Read the model definition and answer for the solid it produces. Units are mm, in the model's axes. A direction names the side the tool comes from. Give positions to 0.01 mm unless a question says otherwise; leave off trailing zeros. Order: outer loops, then holes, each group sorted by start corner. A loop starts at its lowest first (then second) coordinate and runs counter-clockwise, first axis right, second up. Notation, with made-up numbers: (30, 68) - (75, 68) arc R24 cw to (75, 90) - close; hole circle Ø1 at (-9, 30). An arc over 180 degrees is marked (long way). Use a Markdown table: item, result. Add a question column.
1. Consider L1, parallel to Y at x = 4.4, z = 0; L2, parallel to X at y = 9.75, z = 2.5; L3, parallel to Y at x = 13.6, z = 0. Determine where each line is inside the solid, lowest interval first.
2. A cutting plane is placed at B-B on x = -112.5. Determine the outline of the cut face in (y, z).
3. For a pull along X with two mould halves and no side action, classify faces 6 (the cylindrical face through (2.769, 12.082, 5.323)), 7 (the cylindrical face through (-3.4, 19.3, -0.1)), 8 (the flat face through (12, 10, -4.648)) as released by +X, released by -X, zero draft, split by the parting line, or undercut.
4. Flat-ended cylindrical pins translate along their axes: P1, Ø1.5, axis at x = -109.5, y = 2, coming from the -Z side; P2, Ø0.7, axis at x = 2.5, y = 12.5, coming from the +Z side; P3, Ø3.5, axis at x = -79.5, z = 1, coming from the +Y side; P4, Ø6.5, axis at x = 7.5, z = 0.5, coming from the +Y side. Find the tip coordinate at first contact, or state that the pin passes through.
5. Which of the six approach directions +Z, -Z, +X, -X, +Y, -Y give full straight-line access (tool end or side, diameter ignored) to faces 1 (the flat face through (0, 18.551, 0)), 2 (the flat face through (12, 10, 4.638)), 3 (the flat face through (-75, 9, 5.764)), 4 (the flat face through (11.063, 8, 0)), 5 (the cylindrical face through (13.25, 12.22, -0.26))?
6. A cutting plane is placed at A-A on z = 0. Determine the outline of the cut face in (x, y).
```python
from build123d import *

# Parameters (mm, degrees)
SKETCH1_R               = 6
BOSS_EXTRUDE1_DEPTH     = 20
SKETCH2_R               = 3.4
CUT_EXTRUDE1_DEPTH      = 13.55
SKETCH5_W               = 1.550685087
SKETCH5_H               = 7.184215806
BOSS_EXTRUDE2_DEPTH     = 13.55
SKETCH7_W               = 9.286501956
SKETCH7_H               = 19.909960041
BOSS_EXTRUDE3_DEPTH     = 12.9
SKETCH6_R               = 2
CUT_EXTRUDE2_DEPTH      = 1
CUT_EXTRUDE2_DEPTH_BACK = 13.55
CUT_EXTRUDE3_DEPTH      = 10
CUT_EXTRUDE3_DEPTH_BACK = 10
SKETCH11_W              = 11.756176319
SKETCH11_H              = 18.551417714
BOSS_EXTRUDE4_DEPTH     = 153


with BuildPart() as part:
    # Sketch1 → Boss-Extrude1 (new body)
    with BuildSketch(Plane(origin=(0, 0, 0), x_dir=(1, 0, 0), z_dir=(0, 1, 0))):
        Circle(SKETCH1_R)
    extrude(amount=BOSS_EXTRUDE1_DEPTH)

    # Sketch2 → Cut-Extrude1 (cut)
    with BuildSketch(Plane(origin=(0, 20, 0), x_dir=(1, 0, 0), z_dir=(0, 1, 0))):
        Circle(SKETCH2_R)
    extrude(amount=-CUT_EXTRUDE1_DEPTH, mode=Mode.SUBTRACT)

    # Sketch5 → Boss-Extrude2 (add)
    with BuildSketch(Plane(origin=(0, 18.26, 0), x_dir=(1, 0, 0), z_dir=(0, 1, 0))):
        with Locations((3.375342544, 0.020519704)):
            Rectangle(SKETCH5_W, SKETCH5_H)
    extrude(amount=-BOSS_EXTRUDE2_DEPTH)

    # Sketch7 → Boss-Extrude3 (add)
    with BuildSketch(Plane.ZY.offset(-2.6)):
        with Locations((-0.005218197, 9.954980021)):
            Rectangle(SKETCH7_W, SKETCH7_H)
    extrude(amount=-BOSS_EXTRUDE3_DEPTH)

    # Sketch6 → Cut-Extrude2 (cut, two sides)
    with BuildSketch(Plane.ZY.offset(-2.6)) as cut_extrude2_sk:
        with Locations((0, 10.236925537)):
            Circle(SKETCH6_R)
    extrude(amount=CUT_EXTRUDE2_DEPTH, mode=Mode.SUBTRACT)
    extrude(cut_extrude2_sk.sketch, amount=-CUT_EXTRUDE2_DEPTH_BACK, mode=Mode.SUBTRACT)

    # Sketch9 → Cut-Extrude3 (cut, two sides)
    with BuildSketch(Plane.XY) as cut_extrude3_sk:
        Polygon((11.063430227, 10.236925537), (11.063430227, 5.861925537), (4.943430227, 5.861925537), (4.943430227, 10.236925537), (4.943430227, 14.611925537), (11.063430227, 14.611925537), align=None)
    extrude(amount=CUT_EXTRUDE3_DEPTH, mode=Mode.SUBTRACT)
    extrude(cut_extrude3_sk.sketch, amount=-CUT_EXTRUDE3_DEPTH_BACK, mode=Mode.SUBTRACT)

    # Sketch11 → Boss-Extrude4 (add)
    with BuildSketch(Plane.ZY.offset(-2.6)):
        with Locations((-0.114099009, 9.275708857)):
            Rectangle(SKETCH11_W, SKETCH11_H)
    extrude(amount=BOSS_EXTRUDE4_DEPTH)


solid = part.part
```
Output values:
| question | item | result |
|---|---|---|
| 1 | L1 | 0 to 8.24, 12.24 to 20 |
| 1 | L2 | -150.4 to 4.94, 11.06 to 15.5 |
| 1 | L3 | 0 to 8.24, 12.24 to 19.91 |
| 2 | outline | (0, -5.99) - (18.55, -5.99) - (18.55, 5.76) - (0, 5.76) - close |
| 3 | face 6 | split by the parting line |
| 3 | face 7 | undercut |
| 3 | face 8 | zero draft |
| 4 | P1 | z = -5.99 |
| 4 | P2 | z = 5.76 |
| 4 | P3 | y = 18.55 |
| 4 | P4 | y = 20 |
| 5 | face 1 | +Y |
| 5 | face 2 | +Z, +X, +Y, -Y |
| 5 | face 3 | +Z, -X, +Y, -Y |
| 5 | face 4 | +Z, -Z |
| 5 | face 5 | +X |
| 6 | outline | (-150.4, 0) - (15.5, 0) - (15.5, 8.24) - (11.06, 8.24) - (11.06, 5.86) - (4.94, 5.86) - (4.94, 8.24) - (2.6, 8.24) - (2.6, 12.24) - (4.94, 12.24) - (4.94, 14.61) - (11.06, 14.61) - (11.06, 12.24) - (15.5, 12.24) - (15.5, 19.91) - (6, 19.91) - (6, 20) - (3.4, 20) - (3.4, 19.91) - (2.6, 19.91) - (2.6, 18.55) - (-3.4, 18.55) - (-3.4, 20) - (-6, 20) - (-6, 18.55) - (-150.4, 18.55) - close |
